Here's the drawing with two shaded views (mm, measured from the low corner). I have some questions. Coordinates: 2 decimals unless noted, no trailing zeros. Loops run counter-clockwise (first coordinate to the right, second up) from the corner with the lowest first, then second, coordinate; pieces in that order, holes last. Notation, with made-up numbers: (13.5, -32.75) -> (63.5, -32.75) arc R21 cw to (63.5, -24.75) -> close; hole circle Ø7 at (-8.5, 12). An arc over 180 degrees is marked (long way). Answer as a JSON object with one key per item and string values. Group by question number.
Q1. I want a section at D-D on x = 35. Write out the boundary of the cut face in (y, z).
Q2. I need wall thicknesses on line 1 (Y direction, x = 20, z = 2.4); line 2 (X direction, y = 28.5, z = 3.25); line 3 (Y direction, x = 22, z = 4.25). Which ranges of each line are inside material? Lowest first, please.
Q3. I want a section at A-A on x = 20. Write out the boundary of the cut face in (y, z).
Q4. I want a section at B-B on z = 3. Write out the boundary of the cut face in (x, y).
Q5. I want a section at C-C on y = 96.5. Write out the boundary of the cut face in (x, z), then the cut area to 4 significant figures.
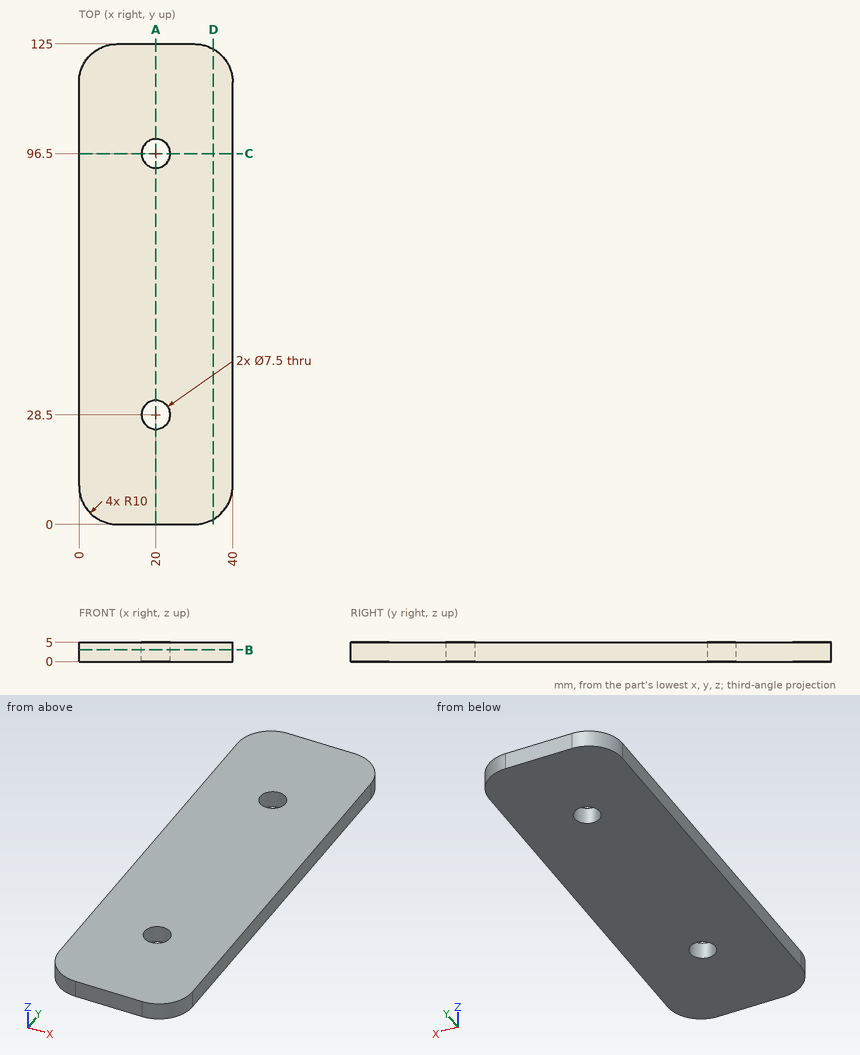
Result set:
{
 "1": {"outline": "(1.34, 0) -> (123.66, 0) -> (123.66, 5) -> (1.34, 5) -> close"},
 "2": {"line 1": "y = 0 to 24.75, 32.25 to 92.75, 100.25 to 125", "line 2": "x = 0 to 16.25, 23.75 to 40", "line 3": "y = 0 to 25.33, 31.67 to 93.33, 99.67 to 125"},
 "3": {"outline": "(0, 0) -> (24.75, 0) -> (24.75, 5) -> (0, 5) -> close; (32.25, 0) -> (92.75, 0) -> (92.75, 5) -> (32.25, 5) -> close; (100.25, 0) -> (125, 0) -> (125, 5) -> (100.25, 5) -> close"},
 "4": {"outline": "(0, 10) arc R10 ccw to (10, 0) -> (30, 0) arc R10 ccw to (40, 10) -> (40, 115) arc R10 ccw to (30, 125) -> (10, 125) arc R10 ccw to (0, 115) -> close; hole circle Ø7.5 at (20, 28.5); hole circle Ø7.5 at (20, 96.5)"},
 "5": {"outline": "(0, 0) -> (16.25, 0) -> (16.25, 5) -> (0, 5) -> close; (23.75, 0) -> (40, 0) -> (40, 5) -> (23.75, 5) -> close", "area": "162.5 mm²"}
}
